Source: CAD feature listing. Evaluate the final solid. Frame: model axes, mm. A direction names the side the tool comes from. Give positions to 0.01 mm unless a question says otherwise; leave off trailing zeros. Order: outer loops, then holes, each group sorted by start corner. A loop starts at its lowest first (then second) coordinate and runs counter-clockwise, first axis right, second up. Notation, with made-up numbers: (-22.75, 37) -> (10.25, 37) arc R33 ccw to (10.25, 71) -> close; hole circle Ø10 at (81, 56). An arc over 180 degrees is marked (long way). Use CSV: the item, a comma, the result in double quotes.
```python
from build123d import *

# Parameters (mm, degrees)
SKETCH1_R           = 57
BOSS_EXTRUDE1_DEPTH = 3
SKETCH2_R           = 15
BOSS_EXTRUDE2_DEPTH = 5
SKETCH3_R           = 13
CUT_EXTRUDE1_DEPTH  = 5
SKETCH4_R           = 10
CUT_EXTRUDE2_DEPTH  = 3
SKETCH6_W           = 5
SKETCH6_H           = 50
CUT_EXTRUDE4_DEPTH  = 5
SKETCH8_R           = 1.5
CUT_EXTRUDE5_DEPTH  = 3
SKETCH9_R           = 4
BOSS_EXTRUDE4_DEPTH = 13
SKETCH11_R          = 1.5
CUT_EXTRUDE6_DEPTH  = 13
CIRPATTERN1_COUNT   = 4


with BuildPart() as part:
    # Sketch1 → Boss-Extrude1 (new body)
    with BuildSketch(Plane.XY):
        Circle(SKETCH1_R)
    extrude(amount=BOSS_EXTRUDE1_DEPTH)

    # Sketch2 → Boss-Extrude2 (add)
    with BuildSketch(Plane(origin=(0, 0, 0), x_dir=(-1, 0, 0), z_dir=(0, 0, -1))):
        Circle(SKETCH2_R)
    extrude(amount=BOSS_EXTRUDE2_DEPTH)

    # Sketch3 → Cut-Extrude1 (cut)
    with BuildSketch(Plane(origin=(0, 0, -5), x_dir=(-1, 0, 0), z_dir=(0, 0, -1))):
        Circle(SKETCH3_R)
    extrude(amount=-CUT_EXTRUDE1_DEPTH, mode=Mode.SUBTRACT)

    # Sketch4 → Cut-Extrude2 (cut)
    with BuildSketch(Plane(origin=(0, 0, 0), x_dir=(-1, 0, 0), z_dir=(0, 0, -1))):
        Circle(SKETCH4_R)
    extrude(amount=-CUT_EXTRUDE2_DEPTH, mode=Mode.SUBTRACT)

    # Sketch6 → Cut-Extrude4 (cut)
    with BuildSketch(Plane(origin=(0, 0, -5), x_dir=(-1, 0, 0), z_dir=(0, 0, -1))):
        Rectangle(SKETCH6_W, SKETCH6_H)
    extrude(amount=-CUT_EXTRUDE4_DEPTH, mode=Mode.SUBTRACT)

    # Sketch8 → Cut-Extrude5 (cut)
    with BuildSketch(Plane(origin=(0, 0, 0), x_dir=(-1, 0, 0), z_dir=(0, 0, -1))):
        with Locations((0, 54)):
            Circle(SKETCH8_R)
        with Locations((54, 0)):
            Circle(SKETCH8_R)
        with Locations((0, -54)):
            Circle(SKETCH8_R)
        with Locations((-54, 0)):
            Circle(SKETCH8_R)
    extrude(amount=-CUT_EXTRUDE5_DEPTH, mode=Mode.SUBTRACT)

    # Sketch9 → Boss-Extrude4 (add)
    with BuildSketch(Plane.XY.offset(3)):
        with Locations((0, 47.37)):
            Circle(SKETCH9_R)
    boss_extrude4 = extrude(amount=BOSS_EXTRUDE4_DEPTH)

    # Sketch11 → Cut-Extrude6 (cut)
    with BuildSketch(Plane.XY.offset(16)):
        with Locations((0, 47.37)):
            Circle(SKETCH11_R)
    cut_extrude6 = extrude(amount=-CUT_EXTRUDE6_DEPTH, mode=Mode.SUBTRACT)

    # CirPattern1: Boss-Extrude4, Cut-Extrude6 ×4 about axis
    cirpattern1_axis = Axis((0, 0, 0), (0, 0, 1))
    for i in range(1, CIRPATTERN1_COUNT):
        add(boss_extrude4.rotate(cirpattern1_axis, i * 360 / CIRPATTERN1_COUNT))
        add(cut_extrude6.rotate(cirpattern1_axis, i * 360 / CIRPATTERN1_COUNT), mode=Mode.SUBTRACT)


solid = part.part
```
1. Section query A-A on z = 4.75. Return loops of the section in (x, y).
Answer below:
outline,"circle Ø8 at (-47.37, 0); circle Ø8 at (0, -47.37); circle Ø8 at (0, 47.37); circle Ø8 at (47.37, 0); hole circle Ø3 at (-47.37, 0); hole circle Ø3 at (0, -47.37); hole circle Ø3 at (0, 47.37); hole circle Ø3 at (47.37, 0)"
2. Section query D-D on y = 54. Return loops of the section in (x, z), plus the area to 3 significant figures.
Answer below:
outline,"(-18.25, 0) -> (-1.5, 0) -> (-1.5, 3) -> (-18.25, 3) -> close; (1.5, 0) -> (18.25, 0) -> (18.25, 3) -> (1.5, 3) -> close"
area,"100 mm²"
3. Ray query, line 1 along X through (y, z) = (0, 11); line 2 along Y through (x, z) = (0, 1.15). Return the intervals inside material, ascending.
Answer below:
line 1,"x = -51.37 to -48.87, -45.87 to -43.37, 43.37 to 45.87, 48.87 to 51.37"
line 2,"y = -57 to -55.5, -52.5 to -10, 10 to 52.5, 55.5 to 57"
4. Pin query (flat end, axial travel): P1, Ø1.6, axis at y = -13.5, z = -1.5, coming from the -X side; P2, Ø1, axis at y = 14, z = -3.5, coming from the -X side; P3, Ø0.9, axis at x = 0.5, y = 47, coming from the +Z side. Return the tip coordinate at first contact, or that it passes through.
Answer below:
P1,"stops at x = -7.98"
P2,"stops at x = -6.54"
P3,"stops at z = 3"
5. Mould query, pull axis Y, two halves, no side actions, for faces 6 (the flat face through (13.4, -1, -5)), 7 (the cylindrical face through (52.654, -21.831, 1.479)), 8 (the cylindrical face through (55.2, -0.9, 1.5)). Classes: released by +Y, released by -Y, zero draft, split by the parting line, or undercut.
Answer below:
face 6,"zero draft"
face 7,"split by the parting line"
face 8,"undercut"
6. Access query for faces 1 (the cylindrical face through (15, 0, -2)), 2 (the cylindrical face through (-50.743, 2.15, 9.409)), 3 (the cylindrical face through (0.325, 52.536, 1.479)), 4 (the flat face through (-47, 2, 16)), 5 (the cylindrical face through (13, 0, -3)). Directions: +Z, -Z, +X, -X, +Y, -Y. A direction counts if a zero-diameter tool reaches every point of the face in a straight line with its end or side. Return the directions, or none.
Answer below:
face 1,"-Z, +X"
face 2,"+Z"
face 3,"+Z, -Z"
face 4,"+Z, +X, -X, +Y, -Y"
face 5,"-Z"
7. Section query C-C on z = -2.75. Return loops of the section in (x, y), plus the area to 3 significant figures.
Answer below:
outline,"(-2.5, -14.79) -> (-2.5, -12.76) arc R13 cw to (-2.5, 12.76) -> (-2.5, 14.79) arc R15 ccw to start; (2.5, -14.79) arc R15 ccw to (2.5, 14.79) -> (2.5, 12.76) arc R13 cw to (2.5, -12.76) -> close"
area,"156 mm²"
8. Section query B-B on x = 0. Count the separate pieces of the cut face and the enclosed holes in it, plus the area to 3 significant figures.
Answer below:
separate pieces,"4"
enclosed holes,"0"
area,"394 mm²"
